from build123d import *

# Parameters (mm, degrees)
F0_W      = 54
F0_H      = 67
F1_DEPTH  = 69.8
F2_W      = 29
F2_H      = 3.3
F3_DEPTH  = 100
F5_DEPTH  = 1.5
F6_R      = 3.15
F7_DEPTH  = 12.5
F9_R      = 20
F10_DEPTH = 1.5
F12_R     = 20
F13_DEPTH = 1.5


with BuildPart() as f1:
    # F0 (on Front) → F1 (new body)
    with BuildSketch(Plane.XZ):
        with Locations((27, 33.5)):
            Rectangle(F0_W, F0_H)
    extrude(amount=F1_DEPTH)

    # F2 (on face) → F3 (cut)
    with BuildSketch(Plane.XY.offset(67)):
        with BuildLine():
            Line((0, -36.5), (10.5455173281, -36.5))
            ThreePointArc((10.5455173281, -36.5), (46, -27), (10.5455173281, -17.5))
            Line((10.5455173281, -17.5), (0, -17.5))
            Line((0, -17.5), (0, -36.5))
        make_face()
        with Locations((14.5, -55.65)):
            Rectangle(F2_W, F2_H)
    extrude(amount=-F3_DEPTH, mode=Mode.SUBTRACT)

    # F4 (on face) → F5 (cut)
    with BuildSketch(Plane.YZ.offset(54)):
        Polygon((-69.8, 67), (-69.8, 59.3613030854), (-41.876951199, 33.8605559632), (-69.8, 8.9028859511), (-69.8, 0), (-66.2085348753, 0), (-35.0458744522, 27.6220695453), (-4.8, 0), (0, 0), (0, 8.3138438763), (-27.9903035886, 33.8760114883), (0, 58.6861561237), (0, 67), (-4.8, 67), (-34.8503444482, 40.1409494059), (-64.2607212067, 67), align=None)
    extrude(amount=-F5_DEPTH, mode=Mode.SUBTRACT)

    # F6 (on face) → F7 (cut)
    with BuildSketch(Plane.XZ.offset(69.8)):
        with Locations((8.3, 33.5)):
            Circle(F6_R)
    extrude(amount=-F7_DEPTH, mode=Mode.SUBTRACT)

    # F9 (on offset) → F10 (cut)
    with BuildSketch(Plane.XY.offset(54.5)):
        with Locations((27, -27)):
            Circle(F9_R)
    extrude(amount=F10_DEPTH, mode=Mode.SUBTRACT)

    # F12 (on offset) → F13 (cut)
    with BuildSketch(Plane(origin=(0, 0, 12.5), x_dir=(1, 0, 0), z_dir=(0, 0, -1))):
        with Locations((27, 27)):
            Circle(F12_R)
    extrude(amount=-F13_DEPTH, mode=Mode.SUBTRACT)


solid = f1.part
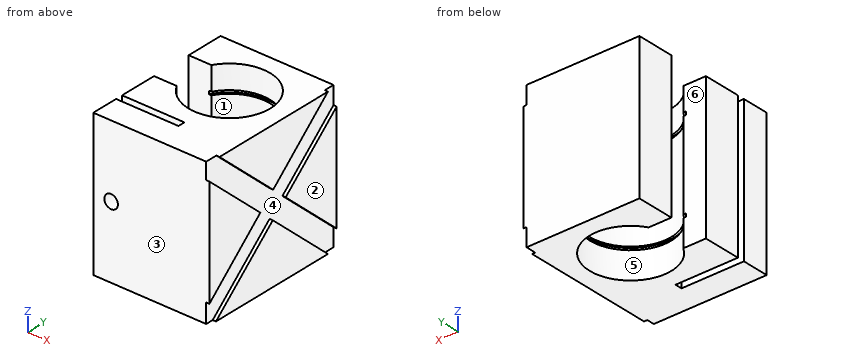
The listing builds one solid part. Answer for the finished solid, in the listing's coordinates (mm). Face numbers are marked on the shaded views. A direction names the side the tool comes from. Give positions to 0.01 mm unless a question says otherwise; leave off trailing zeros. Write each loop counter-clockwise with the first axis right and the second up, starting at its lowest first coordinate (ties: lowest second). Pieces come first, ordered by that corner, then holes.
1) Section B-B (x = 27) is taken. Write down the section's boundary in (y, z), and give its area (3 significant figures).
2) Section C-C (z = 32) is taken. Write down the section's boundary in (x, y).
3) Section A-A (x = 8.3) is taken. Write down the section's boundary in (y, z).
4) For a pull along X with two mould halves and no side action, classify the marked faces 1, 2 and 3 as pulls with the +X half, pulls with the -X half, needs draft (parallel to the pull), parting line crosses it, or undercut.
5) Find the intervals of material crossed by L1, parallel to Y at x = 7, z = 59.5; L2, parallel to Z at x = 8, y = -67; L3, parallel to X at y = -57, z = 33, in increasing order.
6) A tool of negligible diameter and unlimited length cuts with its end or side. For the marked faces 4, 5 and 6, from which of +Z, -Z, +X, -X, +Y, -Y can it reach the whole face along a straight path? Write none if from no direction.
Response:
1. outline: (-69.8, 0) - (-57.3, 0) - (-57.3, 67) - (-69.8, 67) - close; (-54, 0) - (-46, 0) - (-46, 12.5) - (-47, 12.5) - (-47, 14) - (-46, 14) - (-46, 54.5) - (-47, 54.5) - (-47, 56) - (-46, 56) - (-46, 67) - (-54, 67) - close; (-8, 0) - (0, 0) - (0, 67) - (-8, 67) - (-8, 56) - (-7, 56) - (-7, 54.5) - (-8, 54.5) - (-8, 14) - (-7, 14) - (-7, 12.5) - (-8, 12.5) - close
1. area: 1,900 mm2
2. outline: (0, -69.8) - (5.53, -69.8) - (5.53, -57.3) - (0, -57.3) - close; (0, -54) - (29, -54) - (29, -57.3) - (11.07, -57.3) - (11.07, -69.8) - (54, -69.8) - (54, -43.96) - (52.5, -43.96) - (52.5, -25.94) - (54, -25.94) - (54, 0) - (0, 0) - (0, -17.5) - (10.55, -17.5) arc R19 cw (long way) to (10.55, -36.5) - (0, -36.5) - close
3. outline: (-69.8, 0) - (-57.3, 0) - (-57.3, 30.35) - (-69.8, 30.35) - close; (-69.8, 36.65) - (-57.3, 36.65) - (-57.3, 67) - (-69.8, 67) - close; (-54, 0) - (-36.5, 0) - (-36.5, 67) - (-54, 67) - close; (-17.5, 0) - (0, 0) - (0, 67) - (-17.5, 67) - close
4. face 1: undercut
4. face 2: pulls with the +X half
4. face 3: needs draft
5. L1: y = -69.8 to -57.3, -54 to -36.5, -17.5 to 0
5. L2: z = 0 to 30.36, 36.64 to 67
5. L3: x = 29 to 54
6. face 4: +X
6. face 5: +Z, -Z
6. face 6: +Z, -Z, -X
